Here's the drawing with two shaded views (mm, measured from the low corner). I have some questions. Coordinates: 2 decimals unless noted, no trailing zeros. Loops run counter-clockwise (first coordinate to the right, second up) from the corner with the lowest first, then second, coordinate; pieces in that order, holes last.
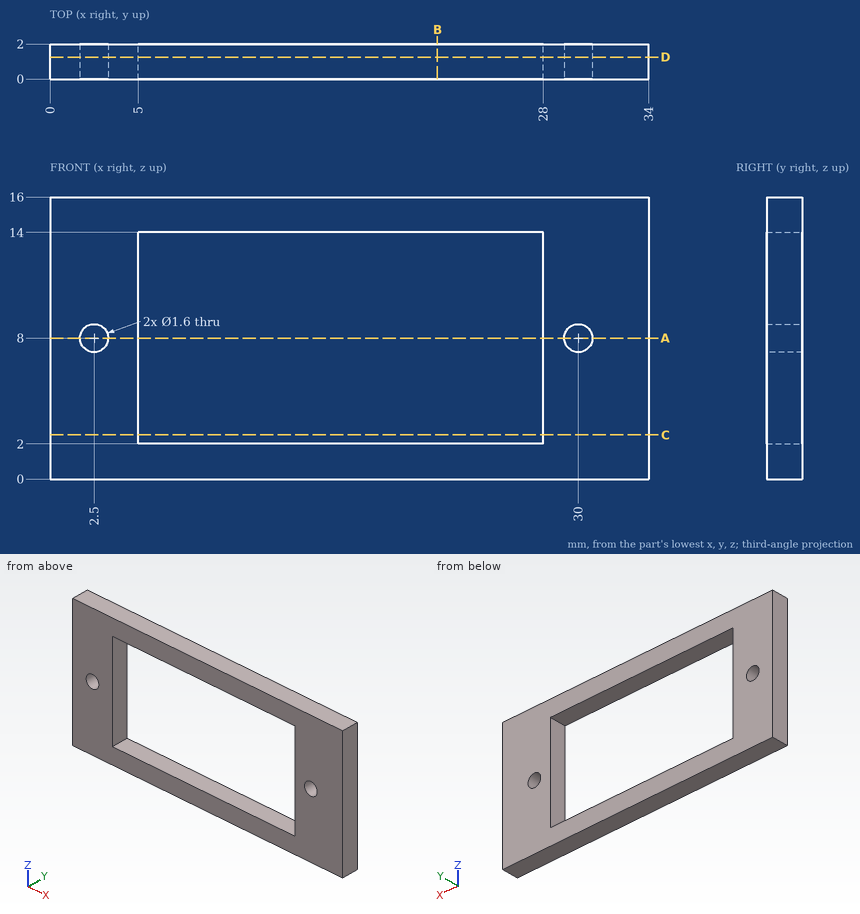
(1) I'm going to push a flat-ended pin straight in: pin 1 (2.5 mm diameter, centred on x = 2.5, z = 8, fed in from -Y). Where does the tip first touch, or does it pass through?
Check values:
pin 1: stops at y = 0
(2) I want a section at A-A on z = 8. Write out the boundary of the cut face in (x, y).
Check values:
outline: (0, 0) - (1.7, 0) - (1.7, 2) - (0, 2) - close; (3.3, 0) - (5, 0) - (5, 2) - (3.3, 2) - close; (28, 0) - (29.2, 0) - (29.2, 2) - (28, 2) - close; (30.8, 0) - (34, 0) - (34, 2) - (30.8, 2) - close
(3) If I drill on probe 1 along X at (y, z) = (0.55, 8); probe 2 along X at (y, z) = (1.95, 7.5); probe 3 along X at (y, z) = (1.2, 6.75), over which ranges is the centre line in solid material (lowest first)?
Check values:
probe 1: x = 0 to 1.7, 3.3 to 5, 28 to 29.2, 30.8 to 34
probe 2: x = 0 to 1.88, 3.12 to 5, 28 to 29.38, 30.62 to 34
probe 3: x = 0 to 5, 28 to 34
(4) I want a section at D-D on y = 1.25. Write out the boundary of the cut face in (x, z).
Check values:
outline: (0, 0) - (34, 0) - (34, 16) - (0, 16) - close; hole circle Ø1.6 at (2.5, 8); hole (5, 2) - (28, 2) - (28, 14) - (5, 14) - close; hole circle Ø1.6 at (30, 8)
(5) I want a section at B-B on x = 22. Write out the boundary of the cut face in (y, z).
Check values:
outline: (0, 0) - (2, 0) - (2, 2) - (0, 2) - close; (0, 14) - (2, 14) - (2, 16) - (0, 16) - close
(6) I want a section at C-C on z = 2.5. Write out the boundary of the cut face in (x, y).
Check values:
outline: (0, 0) - (5, 0) - (5, 2) - (0, 2) - close; (28, 0) - (34, 0) - (34, 2) - (28, 2) - close
